Geometry check sheet. Reference: the model listing, model coordinates, mm. Face numbers are marked on the shaded views. A direction names the side the tool comes from. Round coordinates to 2 decimals unless told otherwise and drop trailing zeros. Write each loop counter-clockwise with the first axis right and the second up, starting at its lowest first coordinate (ties: lowest second). Pieces come first, ordered by that corner, then holes. Notation, with made-up numbers: (-15.75, 56) -> (-11.75, 56) arc R25 cw to (-11.75, 82) -> close; hole circle Ø5 at (87.5, 49.25). An arc over 180 degrees is marked (long way). Use a Markdown table: item, result.
```python
from build123d import *

# Parameters (mm, degrees)
SKETCH1_W               = 40
SKETCH1_H               = 40
SKETCH1_W_2             = 38
SKETCH1_H_2             = 38
BOSS_EXTRUDE1_DEPTH     = 15
SKETCH2_W               = 40
SKETCH2_H               = 40
BOSS_EXTRUDE2_DEPTH     = 1.5
SKETCH3_W               = 7.5
SKETCH3_H               = 5
SKETCH3_R               = 1.625
BOSS_EXTRUDE3_DEPTH     = 3.15
SKETCH4_W               = 6
SKETCH4_H               = 10
CUT_EXTRUDE1_DEPTH      = 1
CUT_EXTRUDE1_DEPTH_BACK = 48.5
SKETCH5_W               = 10
SKETCH5_H               = 6
CUT_EXTRUDE2_DEPTH      = 1
CUT_EXTRUDE2_DEPTH_BACK = 41


with BuildPart() as part:
    # Sketch1 → Boss-Extrude1 (new body)
    with BuildSketch(Plane.XY):
        with Locations((20, 20)):
            Rectangle(SKETCH1_W, SKETCH1_H)
        with Locations((20, 20)):
            Rectangle(SKETCH1_W_2, SKETCH1_H_2, mode=Mode.SUBTRACT)
    extrude(amount=BOSS_EXTRUDE1_DEPTH)

    # Sketch2 → Boss-Extrude2 (add)
    with BuildSketch(Plane.XY.offset(15)):
        with Locations((20, 20)):
            Rectangle(SKETCH2_W, SKETCH2_H)
    extrude(amount=BOSS_EXTRUDE2_DEPTH)

    # Sketch3 → Boss-Extrude3 (add)
    with BuildSketch(Plane(origin=(0, 0, 0), x_dir=(-1, 0, 0), z_dir=(0, 0, -1))):
        with Locations((-43.75, 37.5)):
            Rectangle(SKETCH3_W, SKETCH3_H)
        with Locations((-43.75, 37.5)):
            Circle(SKETCH3_R, mode=Mode.SUBTRACT)
    extrude(amount=-BOSS_EXTRUDE3_DEPTH)

    # Sketch4 → Cut-Extrude1 (cut, two sides)
    with BuildSketch(Plane.ZY) as cut_extrude1_sk:
        with Locations((3, 20)):
            Rectangle(SKETCH4_W, SKETCH4_H)
    extrude(amount=CUT_EXTRUDE1_DEPTH, mode=Mode.SUBTRACT)
    extrude(cut_extrude1_sk.sketch, amount=-CUT_EXTRUDE1_DEPTH_BACK, mode=Mode.SUBTRACT)

    # Sketch5 → Cut-Extrude2 (cut, two sides)
    with BuildSketch(Plane.XZ) as cut_extrude2_sk:
        with Locations((20, 3)):
            Rectangle(SKETCH5_W, SKETCH5_H)
    extrude(amount=CUT_EXTRUDE2_DEPTH, mode=Mode.SUBTRACT)
    extrude(cut_extrude2_sk.sketch, amount=-CUT_EXTRUDE2_DEPTH_BACK, mode=Mode.SUBTRACT)


solid = part.part
```
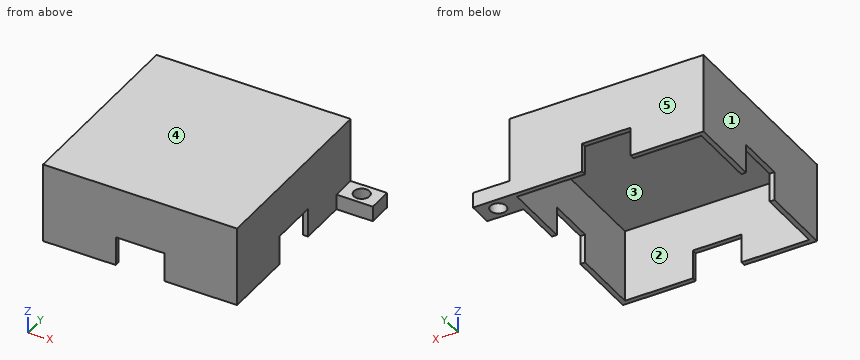
(1) Section check D-D on y = 21.5. Record the cut outline in (x, z), plus the area to 3 significant figures.
A:
| item | result |
|---|---|
| outline | (0, 6) -> (1, 6) -> (1, 15) -> (39, 15) -> (39, 6) -> (40, 6) -> (40, 16.5) -> (0, 16.5) -> close |
| area | 78.0 mm2 |
(2) Section check A-A on x = 43.75. Record the cut outline in (y, z) (3 decimals), plus the area to 3 significant figures.
A:
| item | result |
|---|---|
| outline | (35, 0) -> (35.875, 0) -> (35.875, 3.15) -> (35, 3.15) -> close; (39.125, 0) -> (40, 0) -> (40, 3.15) -> (39.125, 3.15) -> close |
| area | 5.51 mm2 |
(3) Gauge pin test, flat ends, axial feed: pin 1 Ø0.8 at (x, y) = (0.5, 22.5) entering from -Z; pin 2 Ø5 at (y, z) = (15.5, 9.5) entering from +X; pin 3 Ø3 at (x, y) = (34.5, 14.5) entering from -Z. Record the tip position at first contact, or that the pin passes through.
A:
| item | result |
|---|---|
| pin 1 | stops at z = 6 |
| pin 2 | stops at x = 40 |
| pin 3 | stops at z = 15 |
(4) Release check for a two-part mould opening along Y. For the marked faces 3, 4 and 5 record: +Y half, -Y half, draft (parallel to the pull), parting line (faces both ways), or undercut.
A:
| item | result |
|---|---|
| face 3 | undercut |
| face 4 | draft |
| face 5 | +Y half |
(5) Section check B-B on y = 37.5. Record the cut outline in (x, z) (3 decimals).
A:
| item | result |
|---|---|
| outline | (0, 0) -> (1, 0) -> (1, 15) -> (39, 15) -> (39, 0) -> (42.125, 0) -> (42.125, 3.15) -> (40, 3.15) -> (40, 16.5) -> (0, 16.5) -> close; (45.375, 0) -> (47.5, 0) -> (47.5, 3.15) -> (45.375, 3.15) -> close |
(6) Thickness scan on line 1 (Y direction, x = 43.75, z = 2.15) (3 decimals); line 2 (X direction, y = 32, z = 3.5). Record the ranges inside material, lowest first.
A:
| item | result |
|---|---|
| line 1 | y = 35 to 35.875, 39.125 to 40 |
| line 2 | x = 0 to 1, 39 to 40 |
(7) Access from +Z, -Z, +X, -X, +Y, -Y to the whole of each face (thin tool, end or side, straight path). Record for the marked faces 1 and 2.
A:
| item | result |
|---|---|
| face 1 | +Z, -Z, -X, +Y, -Y |
| face 2 | -Z |
(8) Section check C-C on z = 10. Record the cut outline in (x, y).
A:
| item | result |
|---|---|
| outline | (0, 0) -> (40, 0) -> (40, 40) -> (0, 40) -> close; hole (1, 1) -> (39, 1) -> (39, 39) -> (1, 39) -> close |
